from build123d import *

# Parameters (mm, degrees)
PAD005_DEPTH    = 8.5
SKETCH013_R     = 5
PAD006_DEPTH    = 3.1
SKETCH015_R     = 2.8
POCKET005_DEPTH = 10


with BuildPart() as part:
    # Sketch012 (on Face1 of CopyCylinder) → Pad005 (new body)
    with BuildSketch(Plane(origin=(0, 0, 0), x_dir=(1, 0, 0), z_dir=(0, 0, -1))):
        with BuildLine():
            ThreePointArc((-3.25, -1.768474), (0, -3.7), (3.25, -1.768474))
            Line((3.25, -1.768474), (3.25, 1.768474))
            ThreePointArc((3.25, 1.768474), (0, 3.7), (-3.25, 1.768474))
            Line((-3.25, 1.768474), (-3.25, -1.768474))
        make_face()
    extrude(amount=PAD005_DEPTH)

    # Sketch013 (on Face5 of Pad005) → Pad006 (join)
    with BuildSketch(Plane.XY):
        Circle(SKETCH013_R)
    extrude(amount=PAD006_DEPTH)

    # Sketch015 (on Face3 of Pad006) → Pocket005 (cut)
    with BuildSketch(Plane.XY.offset(3.1)):
        Circle(SKETCH015_R)
    extrude(amount=-POCKET005_DEPTH, mode=Mode.SUBTRACT)


solid = part.part
Read the model definition and answer for the solid it produces. Units are mm, in the model's axes. A direction names the side the tool comes from. Round coordinates to 2 decimals unless told otherwise and drop trailing zeros. Write each loop counter-clockwise with the first axis right and the second up, starting at its lowest first coordinate (ties: lowest second). Pieces come first, ordered by that corner, then holes. Notation, with made-up numbers: (46, 86) - (94, 86) arc R20 ccw to (94, 98) - close; hole circle Ø10 at (-40, -39.75). An arc over 180 degrees is marked (long way). Use a Markdown table: item, result.
(1) Straight lines are drawn through the part: line 1 along Z through (x, y) = (1, -4.25); line 2 along Z through (x, y) = (-1, -0.75); line 3 along Y through (x, z) = (0, 0.75). For each, find the intervals that lie inside material, in ascending order. Write a range as [from, to].
Reported:
| item | result |
|---|---|
| line 1 | [0, 3.1] |
| line 2 | [-8.5, -6.9] |
| line 3 | [-5, -2.8], [2.8, 5] |
(2) Which of the six approach directions +Z, -Z, +X, -X, +Y, -Y give full straight-line access (tool end or side, diameter ignored) to faces 1 (the flat face through (2.2, -2.2, 3.1)), 2 (the flat face through (-3.25, 0, -4)), 3 (the cylindrical face through (-0.1, 3.7, -4.2)), 4 (the flat face through (3.25, 0, -4))?
Reported:
| item | result |
|---|---|
| face 1 | +Z, +X, -X, +Y, -Y |
| face 2 | -Z, -X, +Y, -Y |
| face 3 | -Z, +Y |
| face 4 | -Z, +X, +Y, -Y |
(3) The part is cut by section B-B (x = 0). Write down the section's boundary in (y, z).
Reported:
| item | result |
|---|---|
| outline | (-5, 0) - (-3.7, 0) - (-3.7, -8.5) - (3.7, -8.5) - (3.7, 0) - (5, 0) - (5, 3.1) - (2.8, 3.1) - (2.8, -6.9) - (-2.8, -6.9) - (-2.8, 3.1) - (-5, 3.1) - close |
(4) The part is cut by section C-C (y = 0). Write down the section's boundary in (x, z).
Reported:
| item | result |
|---|---|
| outline | (-5, 0) - (-3.25, 0) - (-3.25, -8.5) - (3.25, -8.5) - (3.25, 0) - (5, 0) - (5, 3.1) - (2.8, 3.1) - (2.8, -6.9) - (-2.8, -6.9) - (-2.8, 3.1) - (-5, 3.1) - close |
(5) The part is cut by section A-A (z = -6.75). Write down the section's boundary in (x, y).
Reported:
| item | result |
|---|---|
| outline | (-3.25, -1.77) arc R3.7 ccw to (3.25, -1.77) - (3.25, 1.77) arc R3.7 ccw to (-3.25, 1.77) - close; hole circle Ø5.6 at (0, 0) |
(6) The mould has two halves that part along Y. Classify faces 5 (the cylindrical face through (-2.8, 0.1, -1.8)), 6 (the flat face through (0, 0, -6.9)), 7 (the cylindrical face through (0.1, -3.7, -4.2)), 8 (the flat face through (-3.403, 0.07, 0)): released by +Y, released by -Y, zero draft, split by the parting line, or undercut.
Reported:
| item | result |
|---|---|
| face 5 | undercut |
| face 6 | undercut |
| face 7 | released by -Y |
| face 8 | zero draft |
(7) Each of these flat-tipped pins is pushed along its axis until it touches: pin 1 Ø5 at (x, z) = (-3, -7) entering from +Y; pin 2 Ø1.8 at (y, z) = (0.5, -4) entering from -X; pin 3 Ø3 at (x, y) = (1, 0.5) entering from +Z. Where does it stop, or does it pass through?
Reported:
| item | result |
|---|---|
| pin 1 | y = 3.67 |
| pin 2 | x = -3.25 |
| pin 3 | z = -6.9 |
(8) The part is cut by section D-D (z = 2). Write down the section's boundary in (x, y).
Reported:
| item | result |
|---|---|
| outline | circle Ø10 at (0, 0); hole circle Ø5.6 at (0, 0) |
